Design review of the part built by this model. Coordinates are the model's own, in mm. A direction names the side the tool comes from. Coordinates: 2 decimals unless noted, no trailing zeros. Loops run counter-clockwise (first coordinate to the right, second up) from the corner with the lowest first, then second, coordinate; pieces in that order, holes last. Notation, with made-up numbers: (-31, -40) -> (-25, -40) arc R22 cw to (-25, -5) -> close; hole circle Ø8 at (75.25, 12). An arc over 180 degrees is marked (long way). Use a Markdown table: item, result. Add a question column.
Q1. For faces 1 (the face through (26, 1.5, 173)), 2 (the face through (0.7, 45.9, 329.3)), 3 (the face through (0, 14, 172)), list the 3-axis set-ups (+Z, -Z, +X, -X, +Y, -Y) from which the entire face can be reached by the end or side of a thin tool; tool diameter is ignored.
Q2. For probe 1 along Y at (x, z) = (39, 219), list the stretches that pass through material, from the lowest coordinate up.
Q3. Take a section at A-A on z = 319. Write out the cut boundary in (x, y), plus the area to 3 significant figures.
Q4. Draft analysis for pull direction Z (two halves, no side actions). For faces 4 (the face through (0.7, 45.7, 20.1)), 5 (the face through (26, 0, 172)), state which applies: pulls with the +Z half, pulls with the -Z half, needs draft (parallel to the pull), parting line crosses it, or undercut.
Q5. Clearance check with flat-ended pins moving along their axes: pin 1 Ø1 at (y, z) = (15, 207) entering from +X; pin 2 Ø6 at (x, z) = (36.5, 101) entering from +Y; pin 3 Ø1.6 at (x, y) = (16.5, 0.5) entering from -Z. State where each tip first meets the part, or that it passes through.
Q6. Take a section at B-B on x = 7. Write out the cut boundary in (y, z), plus the area to 3 significant figures.
Q7. Take a section at C-C on y = 5. Write out the cut boundary in (x, z).
Q8. Take a section at D-D on z = 282.5. Write out the cut boundary in (x, y).
from build123d import *

# Parameters (mm, degrees)
SALIENTE_EXTRUIR1_DEPTH = 349.2
CROQUIS2_R              = 4
CORTAR_EXTRUIR1_DEPTH   = 2
CROQUIS4_W              = 49.3
CROQUIS4_H              = 25.4
CORTAR_EXTRUIR2_DEPTH   = 2
CROQUIS5_W              = 299.2
CROQUIS5_H              = 30
CORTAR_EXTRUIR3_DEPTH   = 2
CHAFL_N1_SIZE           = 10


with BuildPart() as part:
    # Croquis1 → Saliente-Extruir1 (new body)
    with BuildSketch(Plane.XY):
        Polygon((0, 0), (0, 50.8), (1.5, 50.8), (1.5, 1.5), (50.8, 1.5), (50.8, 0), align=None)
    extrude(amount=SALIENTE_EXTRUIR1_DEPTH)

    # Croquis2 → Cortar-Extruir1 (cut)
    with BuildSketch(Plane.ZY):
        with Locations((126.6, 25.4)):
            Circle(CROQUIS2_R)
        with Locations((222.6, 25.4)):
            Circle(CROQUIS2_R)
        with Locations((30.6, 25.4)):
            Circle(CROQUIS2_R)
        with Locations((318.6, 25.4)):
            Circle(CROQUIS2_R)
    extrude(amount=-CORTAR_EXTRUIR1_DEPTH, mode=Mode.SUBTRACT)

    # Croquis4 → Cortar-Extruir2 (cut)
    with BuildSketch(Plane(origin=(0, 1.5, 0), x_dir=(1, 0, 0), z_dir=(0, 1, 0))):
        with Locations((26.15, -12.7)):
            Rectangle(CROQUIS4_W, CROQUIS4_H)
        with Locations((26.15, -336.5)):
            Rectangle(CROQUIS4_W, CROQUIS4_H)
    extrude(amount=-CORTAR_EXTRUIR2_DEPTH, mode=Mode.SUBTRACT)

    # Croquis5 → Cortar-Extruir3 (cut)
    with BuildSketch(Plane.ZY):
        with Locations((174.6, 35.8)):
            Rectangle(CROQUIS5_W, CROQUIS5_H)
    extrude(amount=-CORTAR_EXTRUIR3_DEPTH, mode=Mode.SUBTRACT)

    # Chaflán1
    chafl_n1_edges = [part.edges().sort_by_distance(p)[0] for p in [
        (0.75, 50.8, 25),
        (0.75, 50.8, 324.2),
        (0.75, 20.8, 324.2),
        (0.75, 20.8, 25),
    ]]
    chamfer(chafl_n1_edges, length=CHAFL_N1_SIZE)


solid = part.part
Answer list:
| question | item | result |
|---|---|---|
| 1 | face 1 | +Z, -Z, +X, +Y |
| 1 | face 2 | +X, -X, +Y |
| 1 | face 3 | +Z, -Z, -X, +Y, -Y |
| 2 | probe 1 | 0 to 1.5 |
| 3 | outline | (0, 0) -> (50.8, 0) -> (50.8, 1.5) -> (1.5, 1.5) -> (1.5, 25.6) -> (0, 25.6) -> close |
| 3 | area | 112 mm² |
| 4 | face 4 | undercut |
| 4 | face 5 | needs draft |
| 5 | pin 1 | x = 1.5 |
| 5 | pin 2 | y = 1.5 |
| 5 | pin 3 | z = 25.4 |
| 6 | outline | (0, 25.4) -> (1.5, 25.4) -> (1.5, 323.8) -> (0, 323.8) -> close |
| 6 | area | 448 mm² |
| 7 | outline | (0, 0) -> (1.5, 0) -> (1.5, 349.2) -> (0, 349.2) -> close |
| 8 | outline | (0, 0) -> (50.8, 0) -> (50.8, 1.5) -> (1.5, 1.5) -> (1.5, 20.8) -> (0, 20.8) -> close |
